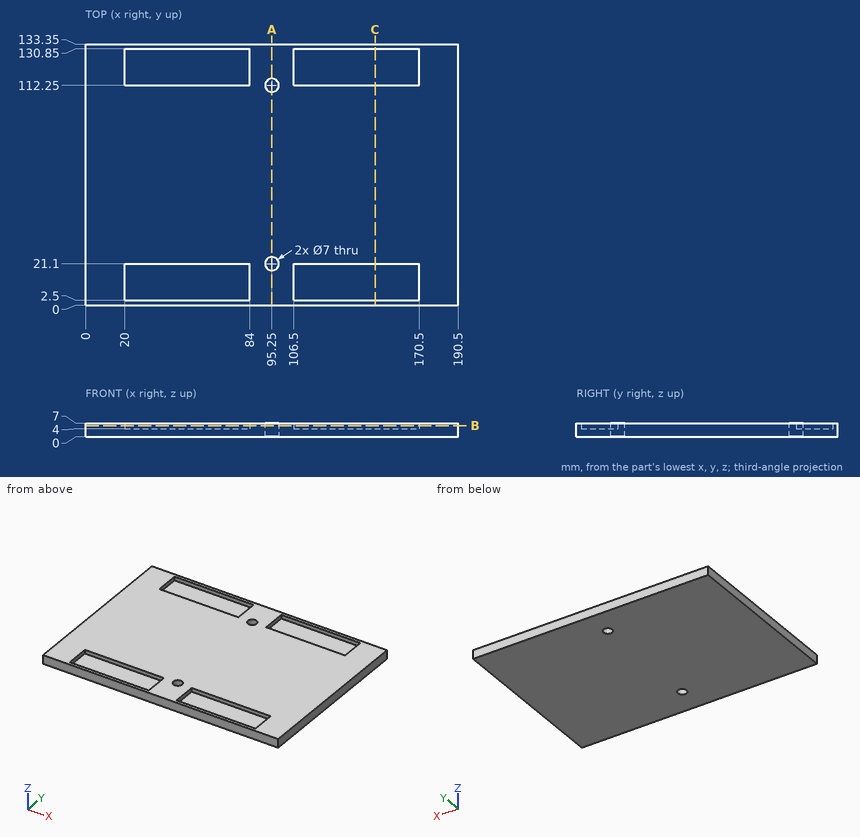
Answer from the drawing. Dimensions are ordinates in mm from the lowest x, y and z of the part. Coordinates: 2 decimals unless noted, no trailing zeros. Order: outer loops, then holes, each group sorted by start corner. A loop starts at its lowest first (then second) coordinate and runs counter-clockwise, first axis right, second up. Notation, with made-up numbers: M 25.25,74 L 64.25,74 A22 cw 64.25,94 Z; hole C 58.5,-11 d3. An arc over 180 degrees is marked long. Put each result on its own line as item: value. Start each with the question number.
Item 1: Section A-A, the plane x = 95.25 is taken. Determine the outline of the cut face in (y, z).
Item 2: Section B-B, the plane z = 5.75 is taken. Determine the outline of the cut face in (x, y), plus the area to 3 significant figures.
Item 3: Consider probe 1 along Y at (x, z) = (120, 5); probe 2 along Y at (x, z) = (95.25, 4.25); probe 3 along Z at (x, y) = (131, 15.5). Determine where each line is inside the solid, lowest interval first. Write a range as [from, to].
Item 4: Given pin 1 Ø3.5 at (y, z) = (118, 5.5) entering from -X, flat-ended and moving along its own axis, determine where the tip first touches the part or whether it passes through.
Item 5: Section C-C, the plane x = 148 is taken. Determine the outline of the cut face in (y, z), plus the area to 3 significant figures.
Computed:
1. outline: M 0,0 L 17.6,0 L 17.6,7 L 0,7 Z; M 24.6,0 L 108.75,0 L 108.75,7 L 24.6,7 Z; M 115.75,0 L 133.35,0 L 133.35,7 L 115.75,7 Z
2. outline: M 0,0 L 190.5,0 L 190.5,133.35 L 0,133.35 Z; hole M 20,2.5 L 84,2.5 L 84,21.1 L 20,21.1 Z; hole M 20,112.25 L 84,112.25 L 84,130.85 L 20,130.85 Z; hole C 95.25,21.1 d7; hole C 95.25,112.25 d7; hole M 106.5,2.5 L 170.5,2.5 L 170.5,21.1 L 106.5,21.1 Z; hole M 106.5,112.25 L 170.5,112.25 L 170.5,130.85 L 106.5,130.85 Z
2. area: 20,600 mm2
3. probe 1: y = [0, 2.5], [21.1, 112.25], [130.85, 133.35]
3. probe 2: y = [0, 17.6], [24.6, 108.75], [115.75, 133.35]
3. probe 3: z = [0, 4]
4. pin 1: stops at x = 0
5. outline: M 0,0 L 133.35,0 L 133.35,7 L 130.85,7 L 130.85,4 L 112.25,4 L 112.25,7 L 21.1,7 L 21.1,4 L 2.5,4 L 2.5,7 L 0,7 Z
5. area: 822 mm2
